Geometry check sheet. Reference: the model listing, model coordinates, mm. Face numbers are marked on the shaded views. A direction names the side the tool comes from. Give positions to 0.01 mm unless a question says otherwise; leave off trailing zeros. Write each loop counter-clockwise with the first axis right and the second up, starting at its lowest first coordinate (ties: lowest second). Pieces come first, ordered by that corner, then holes. Notation, with made-up numbers: (77.25, 81.5) -> (136.25, 81.5) arc R9 ccw to (136.25, 98.5) -> close; hole circle Ø6 at (-22.75, 75). An arc over 180 degrees is marked (long way). One line per item, written item: value.
from build123d import *

# Parameters (mm, degrees)
BOSS_EXTRUDE1_DEPTH = 12.7
SKETCH4_R           = 2.54
CUT_EXTRUDE3_DEPTH  = 37.189429396
CUT_EXTRUDE4_DEPTH  = 5.08


with BuildPart() as part:
    # Sketch3 → Boss-Extrude1 (new body)
    with BuildSketch(Plane(origin=(0, 0, 0), x_dir=(1, 0, 0), z_dir=(0, 1, 0))):
        with BuildLine():
            Line((-25.4, 7.62), (5.08, 7.62))
            ThreePointArc((5.08, 7.62), (12.7, 0), (5.08, -7.62))
            Line((5.08, -7.62), (-25.4, -7.62))
            ThreePointArc((-25.4, -7.62), (-33.02, 0), (-25.4, 7.62))
        make_face()
    extrude(amount=BOSS_EXTRUDE1_DEPTH)

    # Sketch4 → Cut-Extrude3 (cut, through all)
    with BuildSketch(Plane(origin=(0, 12.7, 0), x_dir=(1, 0, 0), z_dir=(0, 1, 0))):
        with Locations(Location((-25.4, 0, 0), (0, 0, 270))):
            Circle(SKETCH4_R)
    extrude(amount=-CUT_EXTRUDE3_DEPTH, mode=Mode.SUBTRACT)

    # Sketch5 → Cut-Extrude4 (cut)
    with BuildSketch(Plane(origin=(0, 12.7, 0), x_dir=(1, 0, 0), z_dir=(0, 1, 0))):
        with BuildLine():
            Line((-11.808123317, -2.469691065), (1.11137089, -4.50000243))
            ThreePointArc((1.11137089, -4.50000243), (11.08000324, 0), (1.11137089, 4.50000243))
            Line((1.11137089, 4.50000243), (-11.808123317, 2.469691065))
            ThreePointArc((-11.808123317, 2.469691065), (-13.92001026, 0), (-11.808123317, -2.469691065))
        make_face()
    extrude(amount=-CUT_EXTRUDE4_DEPTH, mode=Mode.SUBTRACT)


solid = part.part
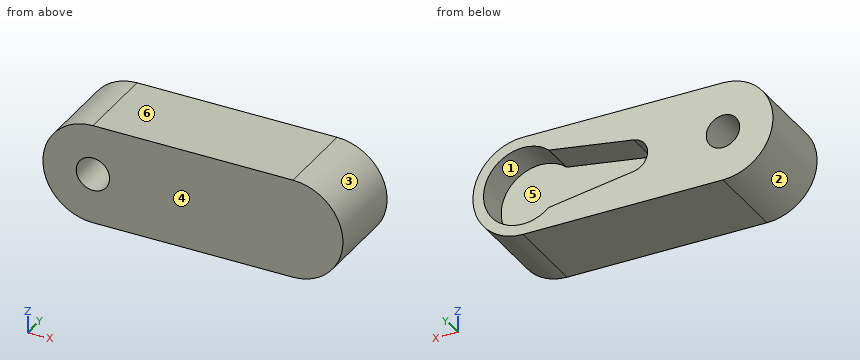
1) Mould release check, pull along X, two halves, no side actions. Record for the marked faces 1, 2, 3 and 4: released by +X, released by -X, zero draft, split by the parting line, or undercut.
Verdict:
face 1: undercut
face 2: released by -X
face 3: released by +X
face 4: zero draft
2) Sectioned sample at B-B on y = 8.25. Record the cut outline in (x, z).
Verdict:
outline: (-25.4, -7.62) -> (5.08, -7.62) arc R7.62 ccw to (5.08, 7.62) -> (-25.4, 7.62) arc R7.62 ccw to start; hole circle Ø5.08 at (-25.4, 0); hole (-11.81, -2.47) -> (1.11, -4.5) arc R6 ccw (long way) to (1.11, 4.5) -> (-11.81, 2.47) arc R2.5 ccw to start
3) Sectioned sample at C-C on y = 3.5. Record the cut outline in (x, z), plus the area to 3 significant figures.
Verdict:
outline: (-25.4, -7.62) -> (5.08, -7.62) arc R7.62 ccw to (5.08, 7.62) -> (-25.4, 7.62) arc R7.62 ccw to start; hole circle Ø5.08 at (-25.4, 0)
area: 627 mm^2
4) Sectioned sample at D-D on x = 3.5. Record the cut outline in (y, z).
Verdict:
outline: (0, -7.62) -> (12.7, -7.62) -> (12.7, -5.79) -> (7.62, -5.79) -> (7.62, 5.79) -> (12.7, 5.79) -> (12.7, 7.62) -> (0, 7.62) -> close
5) Scan lines: probe 1 along X at (y, z) = (12.25, 0); probe 2 along X at (y, z) = (3.5, 0); probe 3 along Z at (x, y) = (5.08, 9.4). Record each from-to range of solid material in increasing order.
Verdict:
probe 1: -33.02 to -27.94, -22.86 to -13.92, 11.08 to 12.7
probe 2: -33.02 to -27.94, -22.86 to 12.7
probe 3: -7.62 to -6, 6 to 7.62
6) Tool access check on the marked faces 5 and 6. Record the directions out of +Z, -Z, +X, -X, +Y, -Y that give a thin tool (end or side, any length) a straight path to the whole face; none if there is none.
Verdict:
face 5: +Y
face 6: +Z, +X, -X, +Y, -Y
7) Sectioned sample at A-A on z = 0. Record the cut outline in (x, y), plus the area to 3 significant figures.
Verdict:
outline: (-33.02, 0) -> (-27.94, 0) -> (-27.94, 12.7) -> (-33.02, 12.7) -> close; (-22.86, 0) -> (12.7, 0) -> (12.7, 12.7) -> (11.08, 12.7) -> (11.08, 7.62) -> (-13.92, 7.62) -> (-13.92, 12.7) -> (-22.86, 12.7) -> close
area: 389 mm^2
